Part model, mm, in its own coordinate system. A direction names the side the tool comes from. Coordinates: 2 decimals unless noted, no trailing zeros. Loops run counter-clockwise (first coordinate to the right, second up) from the corner with the lowest first, then second, coordinate; pieces in that order, holes last. Notation, with made-up numbers: (65.5, -38) - (75.5, -38) arc R30 ccw to (75.5, -14) - close; hole circle Ø6 at (31, -37). An arc over 180 degrees is marked (long way). Use a Markdown table: item, result. Add a question column.
1. Band-saw the part on B-B, the plane z = 0. Give the cut face in (x, y).
2. Wall check: probe 1 along X at (y, z) = (2.5, -17.5); probe 2 along Y at (x, z) = (-39, -4); probe 3 along X at (y, z) = (-1, 0). Give the ranges that are in metal, low to high. Write a range as [from, to].
3. Pull direction Z, two halves, no side cores. Call faces 4 (the flat face through (39, 36, -10)), 5 (the cylindrical face through (37.4, 0.57, -0.28)), 6 (the flat face through (39, 25, -20)), 7 (the cylindrical face through (39.014, 13.102, -3.276)): pulls with the +Z half, pulls with the -Z half, needs draft (parallel to the pull), parting line crosses it, or undercut.
4. Band-saw the part on A-A, the plane y = 34.5. Give the cut face in (x, z), plus the area to 3 significant figures.
5. Drop flat-ended pins along their axis: pin 1 (1.6 mm diameter, centred on x = -39.5, y = 29.5, fed in from -Z); pin 2 (4.5 mm diameter, centred on x = 12, y = 10, fed in from +Z); pin 3 (12 mm diameter, centred on x = 12, z = -13, fed in from +Y); pin 4 (8 mm diameter, centred on x = -22, z = -3.5, fed in from +Y). Give the stop position or say it passes through.
6. Band-saw the part on D-D, the plane y = 53. Give the cut face in (x, z).
7. 3-axis set-ups, long thin cutter, end or side, ignore diameter. For faces 1 (the flat face through (-39, 36, 10)), 2 (the flat face through (-38, 35, 14)), 3 (the flat face through (40, 34, 14)): which of +Z, -Z, +X, -X, +Y, -Y reach the whole face in a straight line?
8. Band-saw the part on C-C, the plane x = 0. Give the cut face in (y, z), plus the area to 3 significant figures.
from build123d import *

# Parameters (mm, degrees)
EXTRUDE_1_DEPTH     = 20
SKETCH_2_R          = 1.75
CUT_EXTRUDE_1_DEPTH = 10
SKETCH_3_W          = 20
SKETCH_3_H          = 42
CUT_EXTRUDE_2_DEPTH = 107.883113727
SKETCH_4_R          = 2
CUT_EXTRUDE_3_DEPTH = 107.883113727
SKETCH_8_W          = 2
SKETCH_8_H          = 50
EXTRUDE_4_DEPTH     = 25
SKETCH_9_R          = 2.75
CUT_EXTRUDE_4_DEPTH = 8
FILLET_1_R          = 2


with BuildPart() as part:
    # 草图1 → 凸台-拉伸1 (new, symmetric)
    with BuildSketch(Plane.XY):
        Polygon((-38, 0), (38, 0), (38, 68), (40, 68), (40, -2), (-40, -2), (-40, 68), (-38, 68), align=None)
    extrude(amount=EXTRUDE_1_DEPTH, both=True)

    # 草图2 → 切除-拉伸1 (cut)
    with BuildSketch(Plane(origin=(0, 0, 0), x_dir=(1, 0, 0), z_dir=(0, 1, 0))):
        with Locations(Location((0, 7, 0), (0, 0, 270))):
            Circle(SKETCH_2_R)
        with Locations(Location((-7, 0, 0), (0, 0, 270))):
            Circle(SKETCH_2_R)
        with Locations(Location((0, -7, 0), (0, 0, 270))):
            Circle(SKETCH_2_R)
        with Locations(Location((7, 0, 0), (0, 0, 270))):
            Circle(SKETCH_2_R)
    extrude(amount=-CUT_EXTRUDE_1_DEPTH, mode=Mode.SUBTRACT)

    # 草图3 → 切除-拉伸2 (cut, through all)
    with BuildSketch(Plane(origin=(40, 0, 0), x_dir=(0, 0, -1), z_dir=(1, 0, 0))):
        with Locations((0, 36)):
            Rectangle(SKETCH_3_W, SKETCH_3_H)
    extrude(amount=-CUT_EXTRUDE_2_DEPTH, mode=Mode.SUBTRACT)

    # 草图4 → 切除-拉伸3 (cut, through all)
    with BuildSketch(Plane(origin=(40, 0, 0), x_dir=(0, 0, -1), z_dir=(1, 0, 0))):
        with Locations((-4.75, 60.25)):
            Circle(SKETCH_4_R)
        with Locations((4.75, 60.25)):
            Circle(SKETCH_4_R)
        with Locations((-4.75, 11.75)):
            Circle(SKETCH_4_R)
        with Locations((4.75, 11.75)):
            Circle(SKETCH_4_R)
    extrude(amount=-CUT_EXTRUDE_3_DEPTH, mode=Mode.SUBTRACT)

    # 草图8 → 凸台-拉伸4 (add, symmetric)
    with BuildSketch(Plane(origin=(0, 0, 0), x_dir=(0, 0, -1), z_dir=(1, 0, 0))):
        with Locations((21, 23)):
            Rectangle(SKETCH_8_W, SKETCH_8_H)
    extrude(amount=EXTRUDE_4_DEPTH, both=True)

    # 草图9 → 切除-拉伸4 (cut)
    with BuildSketch(Plane.XY.offset(-20)):
        with Locations((12, 10)):
            Circle(SKETCH_9_R)
        with Locations((12, 43)):
            Circle(SKETCH_9_R)
    cut_extrude_4 = extrude(amount=-CUT_EXTRUDE_4_DEPTH, mode=Mode.SUBTRACT)

    # 镜向1: 切除-拉伸4 across plane
    add(cut_extrude_4.mirror(Plane(origin=(0, 0, 0), x_dir=(0, 0, 1), z_dir=(1, 0, 0))), mode=Mode.SUBTRACT)

    # 圆角1
    fillet_1_edges = [part.edges().sort_by_distance(p)[0] for p in [
        (0, -2, -22),
        (0, 0, -20),
        (-38, 0, 0),
        (-40, -2, 0),
        (40, -2, 0),
        (38, 0, 0),
    ]]
    fillet(fillet_1_edges, radius=FILLET_1_R)


solid = part.part
Geometry check:
| question | item | result |
|---|---|---|
| 1 | outline | (-40, 0) arc R2 ccw to (-38, -2) - (-8.75, -2) - (-8.75, 0) - (-36, 0) arc R2 cw to (-38, 2) - (-38, 15) - (-40, 15) - close; (-40, 57) - (-38, 57) - (-38, 68) - (-40, 68) - close; (-5.25, -2) - (5.25, -2) - (5.25, 0) - (-5.25, 0) - close; (8.75, -2) - (38, -2) arc R2 ccw to (40, 0) - (40, 15) - (38, 15) - (38, 2) arc R2 cw to (36, 0) - (8.75, 0) - close; (38, 57) - (40, 57) - (40, 68) - (38, 68) - close |
| 2 | probe 1 | x = [-40, -38], [38, 40] |
| 2 | probe 2 | y = [-1.73, 9.9], [13.6, 15], [57, 58.4], [62.1, 68] |
| 2 | probe 3 | x = [-39.73, -8.75], [-5.25, 5.25], [8.75, 39.73] |
| 3 | face 4 | undercut |
| 3 | face 5 | needs draft |
| 3 | face 6 | pulls with the -Z half |
| 3 | face 7 | undercut |
| 4 | outline | (-40, -20) - (-38, -20) - (-38, -10) - (-40, -10) - close; (-40, 10) - (-38, 10) - (-38, 20) - (-40, 20) - close; (-25, -22) - (25, -22) - (25, -20) - (-25, -20) - close; (38, -20) - (40, -20) - (40, -10) - (38, -10) - close; (38, 10) - (40, 10) - (40, 20) - (38, 20) - close |
| 4 | area | 180 mm^2 |
| 5 | pin 1 | stops at z = -20 |
| 5 | pin 2 | passes through |
| 5 | pin 3 | stops at y = 0.27 |
| 5 | pin 4 | stops at y = 0 |
| 6 | outline | (-40, -20) - (-38, -20) - (-38, -10) - (-40, -10) - close; (-40, 10) - (-38, 10) - (-38, 20) - (-40, 20) - close; (38, -20) - (40, -20) - (40, -10) - (38, -10) - close; (38, 10) - (40, 10) - (40, 20) - (38, 20) - close |
| 7 | face 1 | +X, -X |
| 7 | face 2 | +Z, -Z, +Y |
| 7 | face 3 | +Z, -Z, +X, +Y, -Y |
| 8 | outline | (-2, -20) arc R2 ccw to (0, -22) - (48, -22) - (48, -20) - (2, -20) arc R2 cw to (0, -18) - (0, -8.75) - (-2, -8.75) - close; (-2, -5.25) - (0, -5.25) - (0, 5.25) - (-2, 5.25) - close; (-2, 8.75) - (0, 8.75) - (0, 20) - (-2, 20) - close |
| 8 | area | 166 mm^2 |
